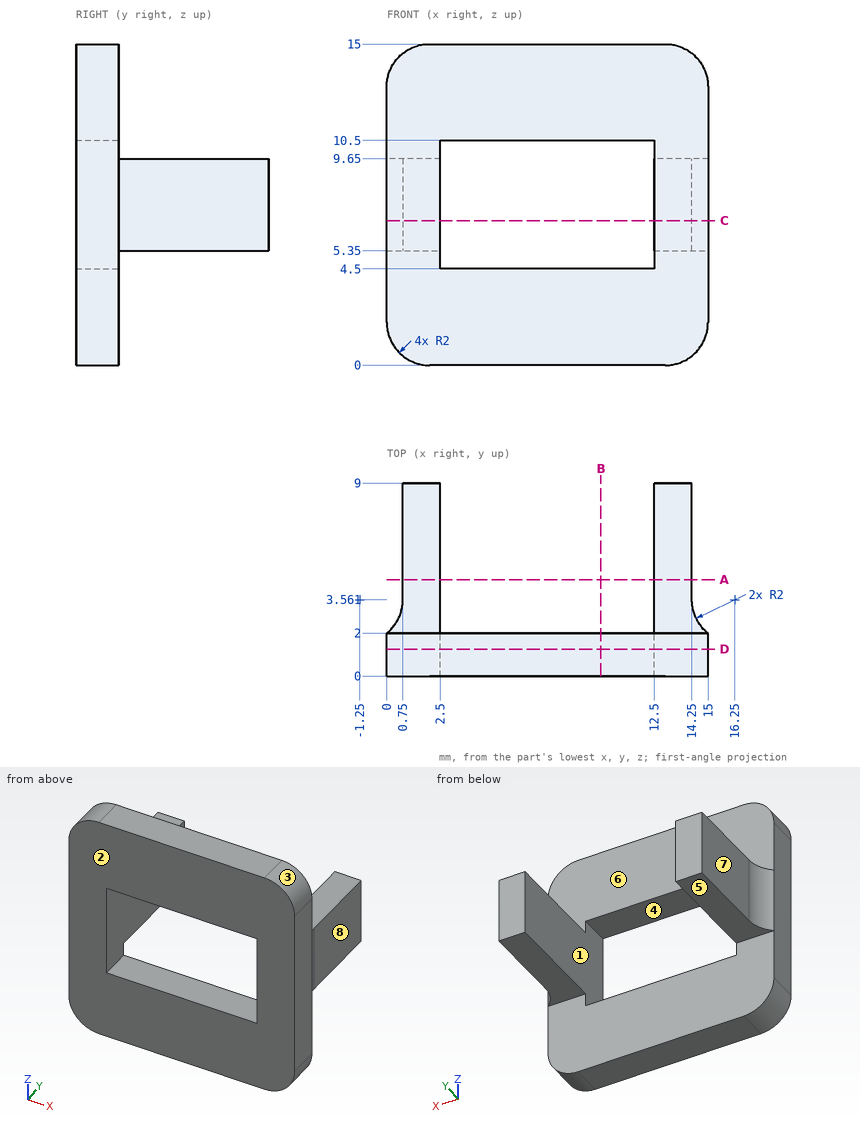
Input: dimensioned drawing with shaded views. Units: mm. Origin: part minimum x, y, z. A direction names the side the tool comes from. Give positions to 0.01 mm unless a question says otherwise; leave off trailing zeros. Order: outer loops, then holes, each group sorted by start corner. A loop starts at its lowest first (then second) coordinate and runs counter-clockwise, first axis right, second up. Notation, with made-up numbers: (-4, -19) -> (21, -19) arc R36 ccw to (21, 17) -> close; hole circle Ø10 at (-39, 50). An arc over 180 degrees is marked (long way). Use one line per item in the form item = value.
1) Line query: probe 1 along X at (y, z) = (3.75, 6.5); probe 2 along Z at (x, y) = (5.5, 1); probe 3 along Y at (x, z) = (12.75, 10.5). Output: solid intervals per line, ascending.
Response values:
probe_1 = 0.75 to 2.5, 12.5 to 14.25
probe_2 = 0 to 4.5, 10.5 to 15
probe_3 = 0 to 2
2) First-contact query: pin 1 Ø3 at (x, y) = (2, 7.5) entering from +Z; pin 2 Ø1 at (y, z) = (3.5, 12.5) entering from -X; pin 3 Ø0.6 at (x, y) = (9.5, 0.5) entering from -Z; pin 4 Ø2 at (x, z) = (6, 12) entering from +Y. Flat tips, straight axial feed; report the tip coordinate or a pass-through.
Response values:
pin_1 = 9.65
pin_2 = through
pin_3 = 0
pin_4 = 2
3) Section A-A, the plane y = 4.5. Return loops of the section in (x, z).
Response values:
outline = (0.75, 5.35) -> (2.5, 5.35) -> (2.5, 9.65) -> (0.75, 9.65) -> close; (12.5, 5.35) -> (14.25, 5.35) -> (14.25, 9.65) -> (12.5, 9.65) -> close
4) Section B-B, the plane x = 10. Return loops of the section in (y, z).
Response values:
outline = (0, 0) -> (2, 0) -> (2, 4.5) -> (0, 4.5) -> close; (0, 10.5) -> (2, 10.5) -> (2, 15) -> (0, 15) -> close
5) Reachability of the marked faces 4, 5, 6, 7 and 8 from +Z, -Z, +X, -X, +Y, -Y: full face, straight path, thin tool, end or side. Return the list, or none.
Response values:
face_4 = +Y, -Y
face_5 = -Z, +X, -X, +Y
face_6 = +Z, +X, -X, +Y
face_7 = +Z, -Z, -X, +Y
face_8 = +Z, -Z, +X, +Y
6) Mould query, pull axis Z, two halves, no side actions, for the marked faces 1, 2 and 3. Classes: pulls with the +Z half, pulls with the -Z half, needs draft (parallel to the pull), parting line crosses it, or undercut.
Response values:
face_1 = undercut
face_2 = needs draft
face_3 = pulls with the +Z half
7) Section D-D, the plane y = 1.25. Return loops of the section in (x, z).
Response values:
outline = (0, 2) arc R2 ccw to (2, 0) -> (13, 0) arc R2 ccw to (15, 2) -> (15, 13) arc R2 ccw to (13, 15) -> (2, 15) arc R2 ccw to (0, 13) -> close; hole (2.5, 4.5) -> (12.5, 4.5) -> (12.5, 10.5) -> (2.5, 10.5) -> close
8) Section C-C, the plane z = 6.75. Return loops of the section in (x, y), and give its area (3 significant figures).
Response values:
outline = (0, 0) -> (2.5, 0) -> (2.5, 9) -> (0.75, 9) -> (0.75, 3.56) arc R2 cw to (0, 2) -> close; (12.5, 0) -> (15, 0) -> (15, 2) arc R2 cw to (14.25, 3.56) -> (14.25, 9) -> (12.5, 9) -> close
area = 35.2 mm^2
